```python
from build123d import *

# Parameters (mm, degrees)
SK_GEARBOX_R              = 18.4
EX_GEARBOX_DEPTH          = 24
SK_MOTOR_R                = 17.4
EX_MOTOR_DEPTH            = 30.7
SK_ENCODER_R              = 17
EX_ENCODER_DEPTH          = 15.4
SK_BUSHING_R              = 6
EX_BUSHING_DEPTH          = 6
SK_SHAFT_R                = 3
EX_SHAFT_DEPTH            = 16
SK_MOUNTHOLES_6XM3_R      = 1.25
CUT_MOUNTHOLES_6XM3_DEPTH = 3


with BuildPart() as part:
    # SK_Gearbox → EX_Gearbox (new body)
    with BuildSketch(Plane(origin=(0, 0, 0), x_dir=(0, 0, -1), z_dir=(1, 0, 0))):
        Circle(SK_GEARBOX_R)
    extrude(amount=-EX_GEARBOX_DEPTH)

    # SK_Motor → EX_Motor (add)
    with BuildSketch(Plane(origin=(-24, 0, 0), x_dir=(0, 0, -1), z_dir=(1, 0, 0))):
        Circle(SK_MOTOR_R)
    extrude(amount=-EX_MOTOR_DEPTH)

    # SK_Encoder → EX_Encoder (add)
    with BuildSketch(Plane(origin=(-54.7, 0, 0), x_dir=(0, 0, -1), z_dir=(1, 0, 0))):
        Circle(SK_ENCODER_R)
    extrude(amount=-EX_ENCODER_DEPTH)

    # SK_Bushing → EX_Bushing (add)
    with BuildSketch(Plane(origin=(0, 0, 0), x_dir=(0, 0, -1), z_dir=(1, 0, 0))):
        with Locations((0, 7)):
            Circle(SK_BUSHING_R)
    extrude(amount=EX_BUSHING_DEPTH)

    # SK_Shaft → EX_Shaft (add)
    with BuildSketch(Plane(origin=(6, 0, 0), x_dir=(0, 0, -1), z_dir=(1, 0, 0))):
        with Locations((0, 7)):
            Circle(SK_SHAFT_R)
    extrude(amount=EX_SHAFT_DEPTH)

    # SK_MountHoles_6xM3 → CUT_MountHoles_6xM3 (cut)
    with BuildSketch(Plane(origin=(0, 0, 0), x_dir=(0, 0, -1), z_dir=(1, 0, 0))):
        with Locations((-15.5, 0)):
            Circle(SK_MOUNTHOLES_6XM3_R)
        with Locations((-7.75, 13.423393759)):
            Circle(SK_MOUNTHOLES_6XM3_R)
        with Locations((7.75, 13.423393759)):
            Circle(SK_MOUNTHOLES_6XM3_R)
        with Locations((15.5, 0)):
            Circle(SK_MOUNTHOLES_6XM3_R)
        with Locations((7.75, -13.423393759)):
            Circle(SK_MOUNTHOLES_6XM3_R)
        with Locations((-7.75, -13.423393759)):
            Circle(SK_MOUNTHOLES_6XM3_R)
    extrude(amount=-CUT_MOUNTHOLES_6XM3_DEPTH, mode=Mode.SUBTRACT)


solid = part.part
```
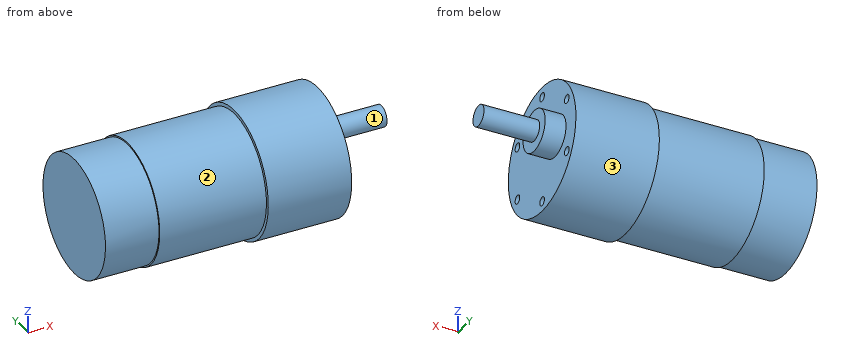
Work out the finished part from the listing and answer in its coordinate system (mm). Face numbers are marked on the shaded views. A direction names the side the tool comes from. Round coordinates to 2 decimals unless told otherwise and drop trailing zeros. Order: outer loops, then holes, each group sorted by start corner. A loop starts at its lowest first (then second) coordinate and runs counter-clockwise, first axis right, second up.
Q1. Given pin 1 Ø2 at (y, z) = (-13.42, -7.75) entering from +X; pin 2 Ø8 at (y, z) = (12, 7.5) entering from +X; pin 3 Ø2 at (y, z) = (-14, -8) entering from +X, each flat-ended and moving along its own axis, determine where each tip first touches the part or whether it passes through.
Solution:
pin 1: stops at x = -3
pin 2: stops at x = 6
pin 3: stops at x = 0
Q2. Find the intervals of material crossed by line 1 along Z through (x, y) = (-2.5, -13); line 2 along X through (y, z) = (9, -3); line 3 along X through (y, z) = (4.5, -9.5), in increasing order.
Solution:
line 1: z = -13.02 to -8.93, -6.57 to 6.57, 8.93 to 13.02
line 2: x = -70.1 to 6
line 3: x = -70.1 to 0
Q3. A tool of negligible diameter and unlimited length cuts with its end or side. For the marked faces 1, 2 and 3, from which of +Z, -Z, +X, -X, +Y, -Y can it reach the whole face along a straight path? Write none if from no direction.
Solution:
face 1: +X
face 2: -X
face 3: +X, -X
Q4. A cutting plane is placed at D-D, the plane y = -16. Determine the outline of the cut face in (x, z).
Solution:
outline: (-70.1, -5.74) - (-54.7, -5.74) - (-54.7, -6.84) - (-24, -6.84) - (-24, -9.09) - (0, -9.09) - (0, 9.09) - (-24, 9.09) - (-24, 6.84) - (-54.7, 6.84) - (-54.7, 5.74) - (-70.1, 5.74) - close
Q5. A cutting plane is placed at A-A, the plane y = 0. Determine the outline of the cut face in (x, z), then the cut area to 3 significant figures.
Solution:
outline: (-70.1, -17) - (-54.7, -17) - (-54.7, -17.4) - (-24, -17.4) - (-24, -18.4) - (0, -18.4) - (0, -16.75) - (-3, -16.75) - (-3, -14.25) - (0, -14.25) - (0, 14.25) - (-3, 14.25) - (-3, 16.75) - (0, 16.75) - (0, 18.4) - (-24, 18.4) - (-24, 17.4) - (-54.7, 17.4) - (-54.7, 17) - (-70.1, 17) - close
area: 2,460 mm2
Q6. A cutting plane is placed at B-B, the plane z = 0. Determine the outline of the cut face in (x, y), then the cut area to 3 significant figures.
Solution:
outline: (-70.1, -17) - (-54.7, -17) - (-54.7, -17.4) - (-24, -17.4) - (-24, -18.4) - (0, -18.4) - (0, 1) - (6, 1) - (6, 4) - (22, 4) - (22, 10) - (6, 10) - (6, 13) - (0, 13) - (0, 18.4) - (-24, 18.4) - (-24, 17.4) - (-54.7, 17.4) - (-54.7, 17) - (-70.1, 17) - close
area: 2,640 mm2
Q7. A cutting plane is placed at C-C, the plane x = -46.5. Determine the outline of the cut face in (y, z), then the cut area to 3 significant figures.
Solution:
outline: circle Ø34.8 at (0, 0)
area: 951 mm2
